from build123d import *

# Parameters (mm, degrees)
BOSS_EXTRUDE1_DEPTH             = 25.4
F_1_8_0_125_DIAMETER_HOLE1_D    = 3.175
F_43_0_089_DIAMETER_HOLE2_D     = 2.2606
F_43_0_089_DIAMETER_HOLE2_DEPTH = 3.175
CUT_EXTRUDE1_REACH              = 44.241
SKETCH8_W                       = 19.05
SKETCH8_H                       = 6.35


with BuildPart() as part:
    # Sketch1 → Boss-Extrude1 (new body)
    with BuildSketch(Plane(origin=(0, 0, 0), x_dir=(1, 0, 0), z_dir=(0, 1, 0))):
        Polygon((0, 0), (0, 25.4), (25.4, 25.4), (25.4, 0), (22.225, 0), (22.225, 22.225), (3.175, 22.225), (3.175, 0), align=None)
    extrude(amount=BOSS_EXTRUDE1_DEPTH)

    # 1/8 (0.125) Diameter Hole1 (through all)
    with Locations(Plane.ZY):
        with Locations((-4.7625, 12.7)):
            Hole(F_1_8_0_125_DIAMETER_HOLE1_D / 2)

    # #43 (0.089) Diameter Hole2
    with Locations(Plane(origin=(25.4, 0, 0), x_dir=(0, 0, -1), z_dir=(1, 0, 0))):
        with Locations((12.7, 19.05), (12.7, 6.35)):
            Hole(F_43_0_089_DIAMETER_HOLE2_D / 2, depth=F_43_0_089_DIAMETER_HOLE2_DEPTH)

    # Sketch8 → Cut-Extrude1 (cut, up to next)
    with BuildSketch(Plane.XY.offset(-22.225), mode=Mode.PRIVATE) as cut_extrude1_sk1:
        with Locations((12.7, 22.225)):
            Rectangle(SKETCH8_W, SKETCH8_H)
    cut_extrude1_tool1 = extrude(cut_extrude1_sk1.sketch, amount=-CUT_EXTRUDE1_REACH, mode=Mode.PRIVATE) & part.part
    # Sketch8 → Cut-Extrude1 (cut, up to next)
    with BuildSketch(Plane.XY.offset(-22.225), mode=Mode.PRIVATE) as cut_extrude1_sk2:
        with Locations((12.7, 3.175)):
            Rectangle(SKETCH8_W, SKETCH8_H)
    cut_extrude1_tool2 = extrude(cut_extrude1_sk2.sketch, amount=-CUT_EXTRUDE1_REACH, mode=Mode.PRIVATE) & part.part
    add(cut_extrude1_tool1.solids().sort_by_distance((12.7, 22.225, -22.225))[0], mode=Mode.SUBTRACT)
    add(cut_extrude1_tool2.solids().sort_by_distance((12.7, 3.175, -22.225))[0], mode=Mode.SUBTRACT)


solid = part.part
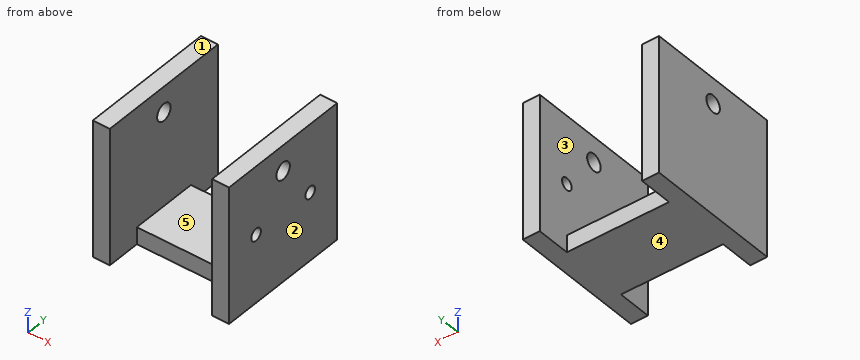
Verification items for the finished model (mm, model axes). Face numbers are marked on the shaded views. A direction names the side the tool comes from. Give positions to 0.01 mm unless a question says otherwise; leave off trailing zeros. Order: outer loops, then holes, each group sorted by start corner. A loop starts at its lowest first (then second) coordinate and runs counter-clockwise, first axis right, second up. Notation, with made-up numbers: M 89,70.25 L 110,70.25 A15 cw 110,88.25 Z; hole C 62.5,71 d7. An arc over 180 degrees is marked long. Answer as a JSON object with one key per item and string values. Group by question number.
1) Access from +Z, -Z, +X, -X, +Y, -Y to the whole of each face (thin tool, end or side, straight path). Record for the marked faces 4 and 5.
2) Depth check by flat-ended pin: pin 1 Ø8 at (x, y) = (16, 7) entering from +Z (3 decimals); pin 2 Ø6 at (y, z) = (22.5, -6) entering from -X; pin 3 Ø3.5 at (x, z) = (9.5, -23.5) entering from +Y; pin 4 Ø2.5 at (x, z) = (11, -24.5) entering from -Y. Enter the tip coordinate at first touch or a pass-through.
3) Cross-section at A-A (z = -2.5). Enter the section's corners in (x, y) (3 decimals).
4) Scan lines: line 1 along Y through (x, z) = (24.7, -12.7); line 2 along X through (y, z) = (21.5, -6.5) (3 decimals); line 3 along Z through (x, y) = (20, 8.75) (3 decimals). Record each from-to range of solid material in increasing order. Write a range as [from, to].
5) Cross-section at B-B (y = 12.7). Enter the section's corners in (x, z) (3 decimals), then the cut area to 3 significant figures.
6) Cross-section at D-D (z = -23.5). Enter the section's corners in (x, y) (3 decimals).
7) Mould release check, pull along X, two halves, no side actions. Record for the marked faces 1, 2 and 3: released by +X, released by -X, zero draft, split by the parting line, or undercut.
8) Cross-section at C-C (z = -12.7). Enter the section's corners in (x, y) (3 decimals).
Result sheet:
{
 "1": {"face 4": "-Z, +X, -X, +Y, -Y", "face 5": "+Z, +Y, -Y"},
 "2": {"pin 1": "stops at z = -22.225", "pin 2": "stops at x = 0", "pin 3": "stops at y = 19.05", "pin 4": "stops at y = 6.35"},
 "3": {"outline": "M 0,0 L 3.175,0 L 3.175,25.4 L 0,25.4 Z; M 22.225,0 L 25.4,0 L 25.4,25.4 L 22.225,25.4 Z"},
 "4": {"line 1": "y = [0, 5.22], [7.48, 17.92], [20.18, 25.4]", "line 2": "x = [0, 3.175], [22.225, 25.4]", "line 3": "z = [-25.4, -22.225]"},
 "5": {"outline": "M 0,-25.4 L 25.4,-25.4 L 25.4,-6.35 L 22.225,-6.35 L 22.225,-22.225 L 3.175,-22.225 L 3.175,-6.35 L 0,-6.35 Z; M 0,-3.175 L 3.175,-3.175 L 3.175,0 L 0,0 Z; M 22.225,-3.175 L 25.4,-3.175 L 25.4,0 L 22.225,0 Z", "area": "202 mm2"},
 "6": {"outline": "M 0,0 L 3.175,0 L 3.175,6.35 L 22.225,6.35 L 22.225,0 L 25.4,0 L 25.4,25.4 L 22.225,25.4 L 22.225,19.05 L 3.175,19.05 L 3.175,25.4 L 0,25.4 Z"},
 "7": {"face 1": "zero draft", "face 2": "released by +X", "face 3": "undercut"},
 "8": {"outline": "M 0,0 L 3.175,0 L 3.175,25.4 L 0,25.4 Z; M 22.225,0 L 25.4,0 L 25.4,5.22 L 22.225,5.22 Z; M 22.225,7.48 L 25.4,7.48 L 25.4,17.92 L 22.225,17.92 Z; M 22.225,20.18 L 25.4,20.18 L 25.4,25.4 L 22.225,25.4 Z"}
}
